The figure shows three views and two pictorial views of one solid part (mm, origin at its lowest corner). Answer the questions. Coordinates: 2 decimals unless noted, no trailing zeros. Loops run counter-clockwise (first coordinate to the right, second up) from the corner with the lowest first, then second, coordinate; pieces in that order, holes last.
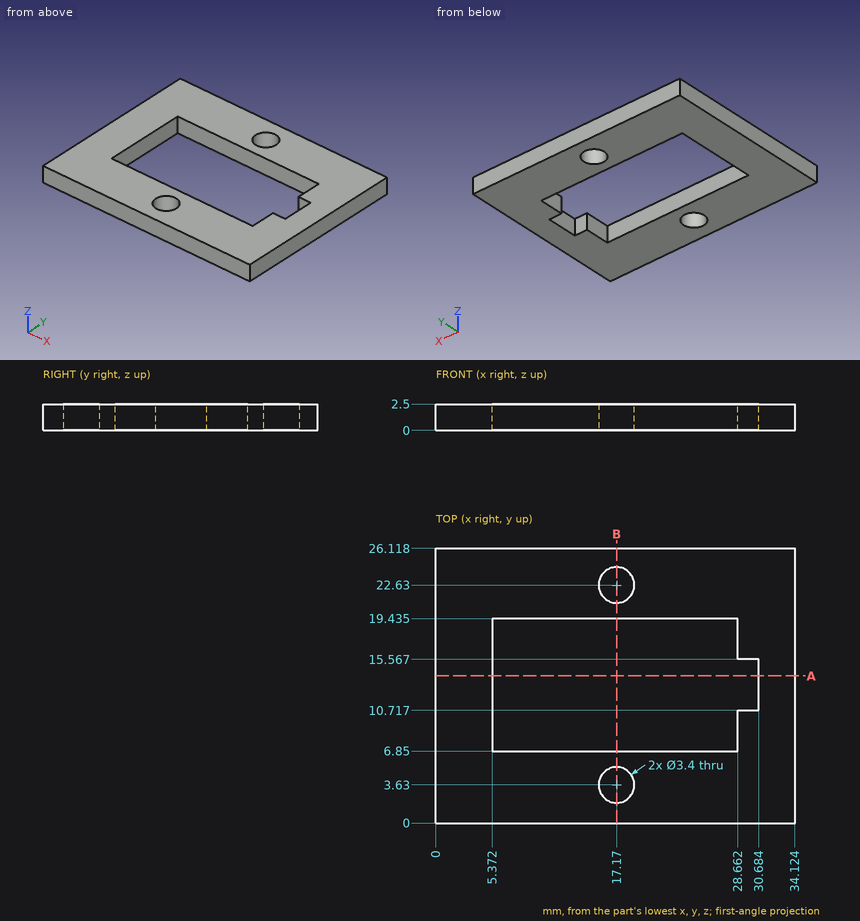
Q1. A cutting plane is placed at A-A (y = 14). Give the vertices of the cut face in (x, z) (1 decimal).
Findings below:
outline: (0, 0) - (5.4, 0) - (5.4, 2.5) - (0, 2.5) - close; (30.7, 0) - (34.1, 0) - (34.1, 2.5) - (30.7, 2.5) - close
Q2. A cutting plane is placed at B-B (x = 17.17). Count the separate pieces of the cut face and the enclosed holes in it.
Findings below:
separate pieces: 4
enclosed holes: 0
Q3. Straight lines are drawn through the part: probe 1 along X at (y, z) = (13.25, 0.5) (1 decimal); probe 2 along X at (y, z) = (9, 1.55) (1 decimal). For each, find the intervals that lie inside material, in ascending order.
Findings below:
probe 1: x = 0 to 5.4, 30.7 to 34.1
probe 2: x = 0 to 5.4, 28.7 to 34.1
